```python
from build123d import *

# Parameters (mm, degrees)
EXTRUDE_2_DEPTH     = 14
FILLET_1_RADIUS     = 7
FILLET_1_LENGTH     = 6.553419282
FILLET_2_RADIUS     = 7
FILLET_2_LENGTH     = 6.553419282
CUT_EXTRUDE_1_REACH = 142.851
SKETCH_2_R          = 2.15
EXTRUDE_3_DEPTH     = 14
FILLET_3_RADIUS     = 7
FILLET_3_LENGTH     = 6
FILLET_4_RADIUS     = 7
FILLET_4_LENGTH     = 6
EXTRUDE_5_REACH     = 144.825
SKETCH_8_R          = 2.5
CUT_EXTRUDE_5_REACH = 145.371
SKETCH_10_R         = 2.15
EXTRUDE_6_REACH     = 144.34
SKETCH_11_R         = 2.5


with BuildPart() as part:
    # Sketch 1 → Extrude 2 (new body)
    with BuildSketch(Plane(origin=(0, 0, 0), x_dir=(1, 0, 0), z_dir=(0, 1, 0))):
        with BuildLine():
            Line((5, 0), (5, 62.718048915))
            ThreePointArc((5, 62.718048915), (4.918829182, 63.989594298), (4.676634468, 65.240497206))
            Line((4.676634468, 65.240497206), (2.323365532, 74.268124597))
            ThreePointArc((2.323365532, 74.268124597), (2.081170818, 75.519027505), (2, 76.790572889))
            Line((2, 76.790572889), (2, 140))
            Line((2, 140), (-4.553419282, 140))
            Line((-4.553419282, 140), (-4.553419282, 76.790572889))
            ThreePointArc((-4.553419282, 76.790572889), (-4.472248464, 75.519027505), (-4.23005375, 74.268124597))
            Line((-4.23005375, 74.268124597), (-1.876784815, 65.240497206))
            ThreePointArc((-1.876784815, 65.240497206), (-1.6345901, 63.989594298), (-1.553419282, 62.718048915))
            Line((-1.553419282, 62.718048915), (-1.553419282, 0))
            Line((-1.553419282, 0), (5, 0))
        make_face()
    extrude(amount=EXTRUDE_2_DEPTH)

    # Fillet 1: full round fillet: the end face becomes a half cylinder, R = half its width
    fillet_1_face = Plane((1.723290359, 7, 0), x_dir=(1, 0, 0), z_dir=(0, 0, 1))  # on the end face: x along it, z out of the body
    fillet_1_slab = fillet_1_face.offset(-FILLET_1_RADIUS / 2) * Box(FILLET_1_LENGTH, 2 * FILLET_1_RADIUS, FILLET_1_RADIUS, mode=Mode.PRIVATE)  # the body's end, R deep
    fillet_1_round = Plane((1.723290359, 7, -7), x_dir=(0, 0, 1), z_dir=(1, 0, 0)) * Cylinder(FILLET_1_RADIUS, FILLET_1_LENGTH, mode=Mode.PRIVATE)  # its axis R under the face
    add(fillet_1_slab - fillet_1_round, mode=Mode.SUBTRACT)

    # Fillet 2: full round fillet: the end face becomes a half cylinder, R = half its width
    fillet_2_face = Plane((-1.276709641, 7, -140), x_dir=(-1, 0, 0), z_dir=(0, 0, -1))  # on the end face: x along it, z out of the body
    fillet_2_slab = fillet_2_face.offset(-FILLET_2_RADIUS / 2) * Box(FILLET_2_LENGTH, 2 * FILLET_2_RADIUS, FILLET_2_RADIUS, mode=Mode.PRIVATE)  # the body's end, R deep
    fillet_2_round = Plane((-1.276709641, 7, -133), x_dir=(0, 0, -1), z_dir=(-1, 0, 0)) * Cylinder(FILLET_2_RADIUS, FILLET_2_LENGTH, mode=Mode.PRIVATE)  # its axis R under the face
    add(fillet_2_slab - fillet_2_round, mode=Mode.SUBTRACT)

    # Sketch 2 → Cut-Extrude 1 (cut, up to next)
    with BuildSketch(Plane(origin=(2, 0, 0), x_dir=(0, 0, -1), z_dir=(1, 0, 0)), mode=Mode.PRIVATE) as cut_extrude_1_sk1:
        with Locations((133, 7)):
            Circle(SKETCH_2_R)
    cut_extrude_1_tool1 = extrude(cut_extrude_1_sk1.sketch, amount=-CUT_EXTRUDE_1_REACH, mode=Mode.PRIVATE) & part.part
    add(cut_extrude_1_tool1.solids().sort_by_distance((2, 7, -133))[0], mode=Mode.SUBTRACT)

    # Sketch 8 → Extrude 5 (add, up to next)
    with BuildSketch(Plane(origin=(-19.553419282, 0, 0), x_dir=(0, 0, -1), z_dir=(1, 0, 0)), mode=Mode.PRIVATE) as extrude_5_sk1:
        with Locations(Location((7, 7, 0), (0, 0, 180))):
            Circle(SKETCH_8_R)
    extrude_5_tool1 = extrude(extrude_5_sk1.sketch, amount=EXTRUDE_5_REACH, mode=Mode.PRIVATE) - part.part
    # Sketch 8 → Extrude 5 (add, up to next)
    with BuildSketch(Plane(origin=(-19.553419282, 0, 0), x_dir=(0, 0, -1), z_dir=(1, 0, 0)), mode=Mode.PRIVATE) as extrude_5_sk2:
        with Locations(Location((57, 7, 0), (0, 0, 180))):
            Circle(SKETCH_8_R)
    extrude_5_tool2 = extrude(extrude_5_sk2.sketch, amount=EXTRUDE_5_REACH, mode=Mode.PRIVATE) - part.part


with BuildPart() as body_2:
    # Sketch 4 → Extrude 3 (new body)
    with BuildSketch(Plane(origin=(0, 0, 0), x_dir=(1, 0, 0), z_dir=(0, 1, 0))):
        with BuildLine():
            Line((-19.553419282, 0), (-25.553419282, 0))
            Line((-25.553419282, 0), (-25.553419282, 62.683862831))
            ThreePointArc((-25.553419282, 62.683862831), (-25.467917646, 63.988746812), (-25.212874842, 65.271316849))
            Line((-25.212874842, 65.271316849), (-22.893963723, 73.928250938))
            ThreePointArc((-22.893963723, 73.928250938), (-22.638920919, 75.210820976), (-22.553419282, 76.515704957))
            Line((-22.553419282, 76.515704957), (-22.553419282, 140))
            Line((-22.553419282, 140), (-16.553419282, 140))
            Line((-16.553419282, 140), (-16.553419282, 76.515704957))
            ThreePointArc((-16.553419282, 76.515704957), (-16.638920919, 75.210820976), (-16.893963723, 73.928250938))
            Line((-16.893963723, 73.928250938), (-19.212874842, 65.271316849))
            ThreePointArc((-19.212874842, 65.271316849), (-19.467917646, 63.988746812), (-19.553419282, 62.683862831))
            Line((-19.553419282, 62.683862831), (-19.553419282, 0))
        make_face()
    extrude(amount=EXTRUDE_3_DEPTH)

    # Fillet 3: full round fillet: the end face becomes a half cylinder, R = half its width
    fillet_3_face = Plane((-19.553419282, 7, -140), x_dir=(-1, 0, 0), z_dir=(0, 0, -1))  # on the end face: x along it, z out of the body
    fillet_3_slab = fillet_3_face.offset(-FILLET_3_RADIUS / 2) * Box(FILLET_3_LENGTH, 2 * FILLET_3_RADIUS, FILLET_3_RADIUS, mode=Mode.PRIVATE)  # the body's end, R deep
    fillet_3_round = Plane((-19.553419282, 7, -133), x_dir=(0, 0, -1), z_dir=(-1, 0, 0)) * Cylinder(FILLET_3_RADIUS, FILLET_3_LENGTH, mode=Mode.PRIVATE)  # its axis R under the face
    add(fillet_3_slab - fillet_3_round, mode=Mode.SUBTRACT)

    # Fillet 4: full round fillet: the end face becomes a half cylinder, R = half its width
    fillet_4_face = Plane((-22.553419282, 7, 0), x_dir=(1, 0, 0), z_dir=(0, 0, 1))  # on the end face: x along it, z out of the body
    fillet_4_slab = fillet_4_face.offset(-FILLET_4_RADIUS / 2) * Box(FILLET_4_LENGTH, 2 * FILLET_4_RADIUS, FILLET_4_RADIUS, mode=Mode.PRIVATE)  # the body's end, R deep
    fillet_4_round = Plane((-22.553419282, 7, -7), x_dir=(0, 0, 1), z_dir=(1, 0, 0)) * Cylinder(FILLET_4_RADIUS, FILLET_4_LENGTH, mode=Mode.PRIVATE)  # its axis R under the face
    add(fillet_4_slab - fillet_4_round, mode=Mode.SUBTRACT)


with BuildPart() as part_1:
    add(part.part)

    add(body_2.part)  # Extrude 5 merges body 2
    add(extrude_5_tool1.solids().sort_by_distance((-19.553419, 7, -7))[0])
    add(extrude_5_tool2.solids().sort_by_distance((-19.553419, 7, -57))[0])

    # Sketch 10 → Cut-Extrude 5 (cut, up to next)
    with BuildSketch(Plane.ZY.offset(22.553419282), mode=Mode.PRIVATE) as cut_extrude_5_sk1:
        with Locations(Location((-133, 7, 0), (0, 0, 180))):
            Circle(SKETCH_10_R)
    cut_extrude_5_tool1 = extrude(cut_extrude_5_sk1.sketch, amount=-CUT_EXTRUDE_5_REACH, mode=Mode.PRIVATE) & part_1.part
    add(cut_extrude_5_tool1.solids().sort_by_distance((-22.553419, 7, -133))[0], mode=Mode.SUBTRACT)

    # Sketch 11 → Extrude 6 (add, up to next)
    with BuildSketch(Plane(origin=(-16.553419282, 0, 0), x_dir=(0, 0, -1), z_dir=(1, 0, 0)), mode=Mode.PRIVATE) as extrude_6_sk1:
        with Locations(Location((103.7, 7, 0), (0, 0, 180))):
            Circle(SKETCH_11_R)
    extrude_6_tool1 = extrude(extrude_6_sk1.sketch, amount=EXTRUDE_6_REACH, mode=Mode.PRIVATE) - part_1.part
    add(extrude_6_tool1.solids().sort_by_distance((-16.553419, 7, -103.7))[0])


solid = part_1.part
```
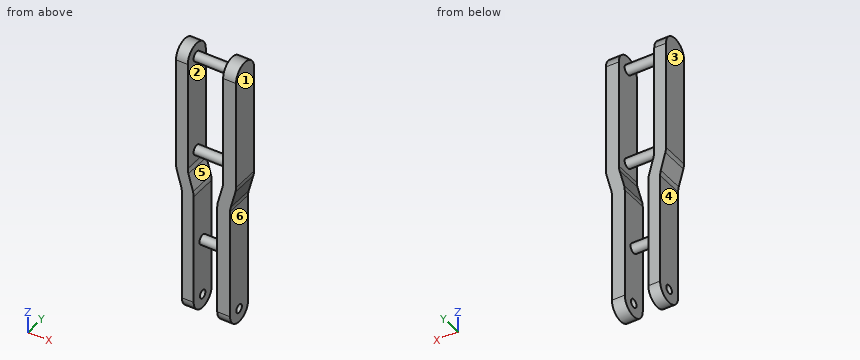
Verification items for the finished model (mm, model axes). Face numbers are marked on the shaded views. A direction names the side the tool comes from. Coordinates: 2 decimals unless noted, no trailing zeros. Order: outer loops, then holes, each group sorted by start corner. A loop starts at its lowest first (then second) coordinate and runs counter-clockwise, first axis right, second up. Notation, with made-up numbers: (-34.5, 35) -> (21.5, 35) arc R25 cw to (21.5, 60) -> close; hole circle Ø10 at (-21.5, -23). An arc over 180 degrees is marked (long way). Answer as CSV lines item,"result". Start each with the question number.
1) Gauge pin test, flat ends, axial feed: pin 1 Ø1.5 at (y, z) = (7, -111) entering from -X; pin 2 Ø5.5 at (y, z) = (7, -133) entering from +X; pin 3 Ø5 at (x, y) = (-9, 8.5) entering from +Z; pin 4 Ø4 at (y, z) = (7, -133) entering from +X. Record the tip position at first contact, or that the pin passes through.
2) Cross-section at A-A, the plane z = -28.5. Record the boundary of the cut face in (x, y), then the cut area to 3 significant figures.
3) Set-up check for the marked faces 4, 5 and 6: record each of +Z, -Z, +X, -X, +Y, -Y from which the full face is reachable in a straight line by a thin tool's end or side.
4) Release check for a two-part mould opening along X. For the marked faces 1, 2 and 3 record: released by +X, released by -X, zero draft, split by the parting line, or undercut.
5) Material ranges on L1, parallel to X at y = 1.25, z = -120; L2, parallel to Y at x = -2, z = -133; L3, parallel to X at y = 12.25, z = -33, recorded low to high. Write a range as [from, to].
6) Cross-section at D-D, the plane x = -9. Record the boundary of the cut face in (y, z), then the cut area to 3 significant figures.
7) Cross-section at C-C, the plane z = -57. Record the boundary of the cut face in (x, y), then the cut area to 3 significant figures.
8) Cross-section at B-B, the plane y = 2.75. Record the boundary of the cut face in (x, z).
Conclusion:
1,pin 1,"stops at x = -22.55"
1,pin 2,"stops at x = 2"
1,pin 3,"stops at z = -4.5"
1,pin 4,"passes through"
2,outline,"(-25.55, 0) -> (-19.55, 0) -> (-19.55, 14) -> (-25.55, 14) -> close; (-1.55, 0) -> (5, 0) -> (5, 14) -> (-1.55, 14) -> close"
2,area,"176 mm²"
3,face 4,"-Z, -X, +Y, -Y"
3,face 5,"+Y, -Y"
3,face 6,"-Z, +X, +Y, -Y"
4,face 1,"released by +X"
4,face 2,"undercut"
4,face 3,"released by -X"
5,L1,"x = [-22.55, -16.55], [-4.55, 2]"
5,L2,"y = [0, 4.85], [9.15, 14]"
5,L3,"x = [-25.55, -19.55], [-1.55, 5]"
6,outline,"circle Ø5 at (7, -103.7); circle Ø5 at (7, -57); circle Ø5 at (7, -7)"
6,area,"58.9 mm²"
7,outline,"(-25.55, 0) -> (-19.55, 0) -> (-19.55, 4.5) -> (-1.55, 4.5) -> (-1.55, 0) -> (5, 0) -> (5, 14) -> (-1.55, 14) -> (-1.55, 9.5) -> (-19.55, 9.5) -> (-19.55, 14) -> (-25.55, 14) -> close"
7,area,"266 mm²"
8,outline,"(-25.55, -62.68) arc R10 ccw to (-25.21, -65.27) -> (-22.89, -73.93) arc R10 cw to (-22.55, -76.52) -> (-22.55, -138.56) -> (-16.55, -138.56) -> (-16.55, -76.52) arc R10 ccw to (-16.89, -73.93) -> (-19.21, -65.27) arc R10 cw to (-19.55, -62.68) -> (-19.55, -1.44) -> (-25.55, -1.44) -> close; (-4.55, -138.56) -> (2, -138.56) -> (2, -76.79) arc R10 cw to (2.32, -74.27) -> (4.68, -65.24) arc R10 ccw to (5, -62.72) -> (5, -1.44) -> (-1.55, -1.44) -> (-1.55, -62.72) arc R10 cw to (-1.88, -65.24) -> (-4.23, -74.27) arc R10 ccw to (-4.55, -76.79) -> close"
